Input: part model. Units: mm. Frame: model coordinates. Face numbers are marked on the shaded views. A direction names the side the tool comes from. Round coordinates to 2 decimals unless told otherwise and drop trailing zeros. Order: outer loops, then holes, each group sorted by start corner. A loop starts at its lowest first (then second) coordinate and runs counter-clockwise, first axis right, second up. Notation, with made-up numbers: (86.25, 12) -> (119.25, 12) arc R20 cw to (119.25, 47) -> close; hole circle Ø8 at (89.5, 63.5). An arc over 180 degrees is marked (long way). Use a Markdown table: item, result.
from build123d import *

# Parameters (mm, degrees)
F0_W     = 635
F0_H     = 457.2
F1_DEPTH = 63.5
F3_DEPTH = 63.501


# Not quite as in the source:
# - a pattern or mirror of a feature is missing from the dataset's text; its kind, count and spacing are read off the source's solid


with BuildPart() as f1:
    # F0 (on Top) → F1 (new body)
    with BuildSketch(Plane.XY):
        with Locations((317.5, -228.6)):
            Rectangle(F0_W, F0_H)
    extrude(amount=-F1_DEPTH)

    # F2 (on Top) → F3 (cut, through all)
    with BuildSketch(Plane.XY):
        Polygon((63.5, -33.6378284982), (0, -42.5621715018), (0, -109.8378284982), (63.5, -118.7621715018), align=None)
        Polygon((63.5, -186.0378284982), (0, -194.9621715018), (0, -262.2378284982), (63.5, -271.1621715018), align=None)
        Polygon((63.5, -338.4378284982), (0, -347.3621715018), (0, -414.6378284982), (63.5, -423.5621715018), align=None)
    f3 = extrude(amount=-F3_DEPTH, mode=Mode.SUBTRACT)

    # F3_copies: F3 across plane
    add(f3.mirror(Plane(origin=(317.5, 0, 0), x_dir=(0, 0, 1), z_dir=(1, 0, 0))), mode=Mode.SUBTRACT)


solid = f1.part
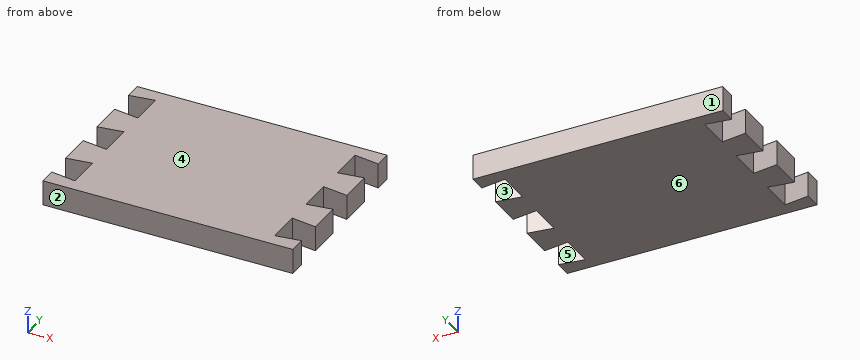
1) Set-up query: the marked faces 5 and 6. Return all of +Z, -Z, +X, -X, +Y, -Y with unobstructed straight access to the full face (end or side cutting, diameter ignored); none if empty.
Answer key:
| item | result |
|---|---|
| face 5 | +Z, -Z |
| face 6 | -Z, +X, -X, +Y, -Y |
2) Ray query, probe 1 along X at (y, z) = (-389.5, -38). Return the intervals inside material, ascending.
Answer key:
| item | result |
|---|---|
| probe 1 | x = 63.5 to 571.5 |
3) Draft query along Y for the marked faces 1, 2, 3 and 4. Return one class per face: released by +Y, released by -Y, zero draft, split by the parting line, or undercut.
Answer key:
| item | result |
|---|---|
| face 1 | released by +Y |
| face 2 | released by -Y |
| face 3 | undercut |
| face 4 | zero draft |
4) Cut plane B-B on y = -405. Return loops of the section in (x, z), and give its area (3 significant figures).
Answer key:
| item | result |
|---|---|
| outline | (63.5, -63.5) -> (571.5, -63.5) -> (571.5, 0) -> (63.5, 0) -> close |
| area | 32,300 mm^2 |
5) Cut plane A-A on z = -55.5. Return loops of the section in (x, y), and give its area (3 significant figures).
Answer key:
| item | result |
|---|---|
| outline | (0, -457.2) -> (635, -457.2) -> (635, -414.64) -> (571.5, -423.56) -> (571.5, -338.44) -> (635, -347.36) -> (635, -262.24) -> (571.5, -271.16) -> (571.5, -186.04) -> (635, -194.96) -> (635, -109.84) -> (571.5, -118.76) -> (571.5, -33.64) -> (635, -42.56) -> (635, 0) -> (0, 0) -> (0, -42.56) -> (63.5, -33.64) -> (63.5, -118.76) -> (0, -109.84) -> (0, -194.96) -> (63.5, -186.04) -> (63.5, -271.16) -> (0, -262.24) -> (0, -347.36) -> (63.5, -338.44) -> (63.5, -423.56) -> (0, -414.64) -> close |
| area | 261,000 mm^2 |
6) Contact query for flat-ended pins moving along their axis: P1, Ø6, axis at y = -62, z = -54.5, coming from the -X side; P2, Ø3, axis at y = -369, z = -21.5, coming from the +X side. Output: stop coordinate, or through.
Answer key:
| item | result |
|---|---|
| P1 | stops at x = 63.5 |
| P2 | stops at x = 571.5 |
